Check sheet for the drawn part. Datum: minimum x, y, z corner. Units: mm. A direction names the side the tool comes from. Give positions to 0.01 mm unless a question says otherwise; leave off trailing zeros. Write each loop counter-clockwise with the first axis right and the second up, starting at its lowest first coordinate (ties: lowest second). Pieces come first, ordered by that corner, then holes.
(1) Cross-section at C-C (z = 7). Record the boundary of the cut face in (x, y), and give its area (3 significant figures).
(2) Cross-section at B-B (y = 7.5). Record the boundary of the cut face in (x, z), and give its area (3 significant figures).
(3) Cross-section at A-A (z = 13.5). Record the boundary of the cut face in (x, y).
(4) Depth check by flat-ended pin: P1, Ø1.5, axis at x = 37, y = 19, coming from the +Z side; P2, Ø11, axis at y = 10.5, z = 16, coming from the -X side; P3, Ø1, axis at x = 54, y = 7.5, coming from the +Z side. Enter the tip coordinate at first touch or a pass-through.
(5) Tool access check on the marked faces 1, 2, 3, 4 and 5. Record the directions out of +Z, -Z, +X, -X, +Y, -Y that give a thin tool (end or side, any length) a straight path to the whole face; none if there is none.
(6) Mould release check, pull along X, two halves, no side actions. Record for the marked faces 6, 7 and 8: +X half, -X half, draft (parallel to the pull), parting line (faces both ways), or undercut.
(7) Thickness scan on line 1 along Y through (x, z) = (61.5, 15); line 2 along X through (y, z) = (6.75, 19); line 3 along X through (y, z) = (11, 8). Record the ranges inside material, lowest first.
(8) Cross-section at D-D (x = 82.5). Record the boundary of the cut face in (y, z), and give its area (3 significant figures).
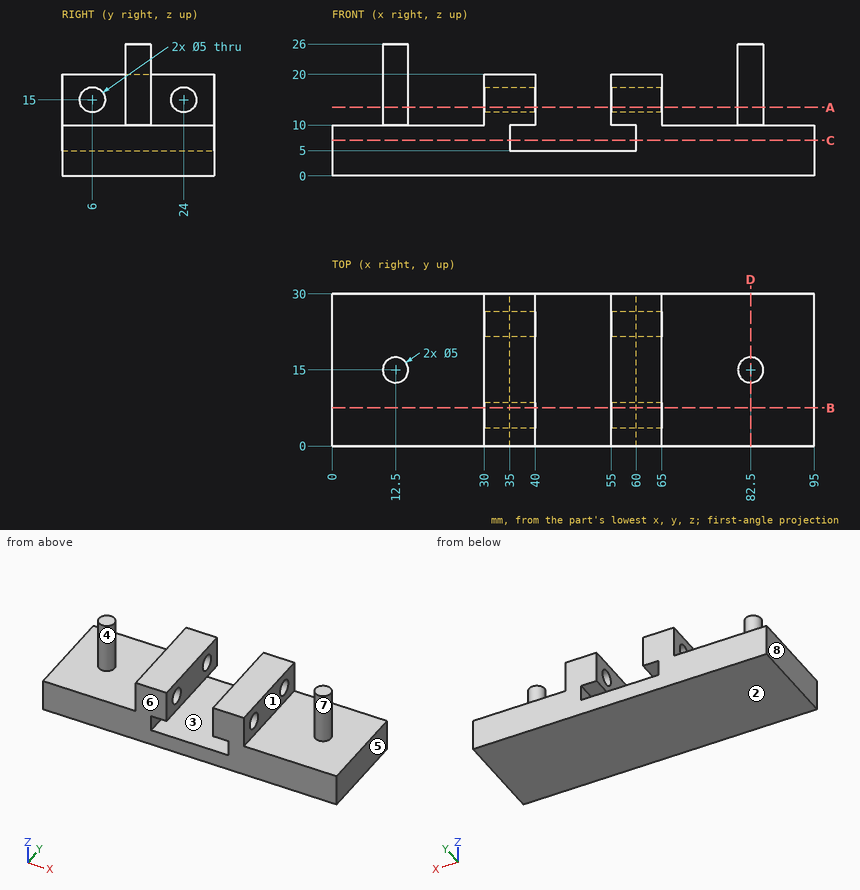
Reply:
1. outline: (0, 0) - (35, 0) - (35, 30) - (0, 30) - close; (60, 0) - (95, 0) - (95, 30) - (60, 30) - close
1. area: 2,100 mm2
2. outline: (0, 0) - (95, 0) - (95, 10) - (65, 10) - (65, 13) - (55, 13) - (55, 10) - (60, 10) - (60, 5) - (35, 5) - (35, 10) - (40, 10) - (40, 13) - (30, 13) - (30, 10) - (0, 10) - close; (30, 17) - (40, 17) - (40, 20) - (30, 20) - close; (55, 17) - (65, 17) - (65, 20) - (55, 20) - close
2. area: 945 mm2
3. outline: circle Ø5 at (12.5, 15); (30, 0) - (40, 0) - (40, 4) - (30, 4) - close; (30, 8) - (40, 8) - (40, 22) - (30, 22) - close; (30, 26) - (40, 26) - (40, 30) - (30, 30) - close; (55, 0) - (65, 0) - (65, 4) - (55, 4) - close; (55, 8) - (65, 8) - (65, 22) - (55, 22) - close; (55, 26) - (65, 26) - (65, 30) - (55, 30) - close; circle Ø5 at (82.5, 15)
4. P1: stops at z = 20
4. P2: stops at x = 10
4. P3: stops at z = 5
5. face 1: +Z, +Y, -Y
5. face 2: -Z, +X, -X, +Y, -Y
5. face 3: +Y, -Y
5. face 4: +Z
5. face 5: +Z, -Z, +X, +Y, -Y
6. face 6: draft
6. face 7: undercut
6. face 8: -X half
7. line 1: y = 0 to 3.5, 8.5 to 21.5, 26.5 to 30
7. line 2: x = 30 to 40, 55 to 65
7. line 3: x = 0 to 35, 60 to 95
8. outline: (0, 0) - (30, 0) - (30, 10) - (17.5, 10) - (17.5, 26) - (12.5, 26) - (12.5, 10) - (0, 10) - close
8. area: 380 mm2
